The drawing under review shows one solid part. Ordinate dimensions are in mm from its lowest x, y, z. A direction names the side the tool comes from. Give positions to 0.01 mm unless a question says otherwise; leave off trailing zeros. Order: outer loops, then holes, each group sorted by start corner. A loop starts at its lowest first (then second) coordinate and runs counter-clockwise, first axis right, second up. Notation, with made-up numbers: (45.5, -33) -> (57.5, -33) arc R20 cw to (57.5, 3) -> close; hole circle Ø3 at (40, 50). An arc over 180 degrees is marked (long way). One line per item, written item: value. Start each with the question number.
1) Consider section A-A (z = 3.25). State the section outline as (x, y) points, plus the area to 3 significant figures.
2) Consider section C-C (z = 17.75). State the section outline as (x, y) points, plus the area to 3 significant figures.
3) Tool access review of the marked faces 1, 2 and 3: name each direction out of +Z, -Z, +X, -X, +Y, -Y from which nothing blocks a thin tool from reaching the whole face with its end or side.
4) Consider section B-B (z = 7). State the section outline as (x, y) points, plus the area to 3 significant figures.
5) For pin 1 (2 mm diameter, centred on y = 2, z = 9.5, fed in from -X), flat-tipped, find the tip position at first contact; note if it passes through.
6) Wall thickness on line 1 along Z through (x, y) = (1.25, 3.25); line 2 along Z through (x, y) = (0.8, 1.9); line 3 along Z through (x, y) = (4, 3.4): over which ranges is each line inside the solid? List them lowest first. Write a range as from..to.
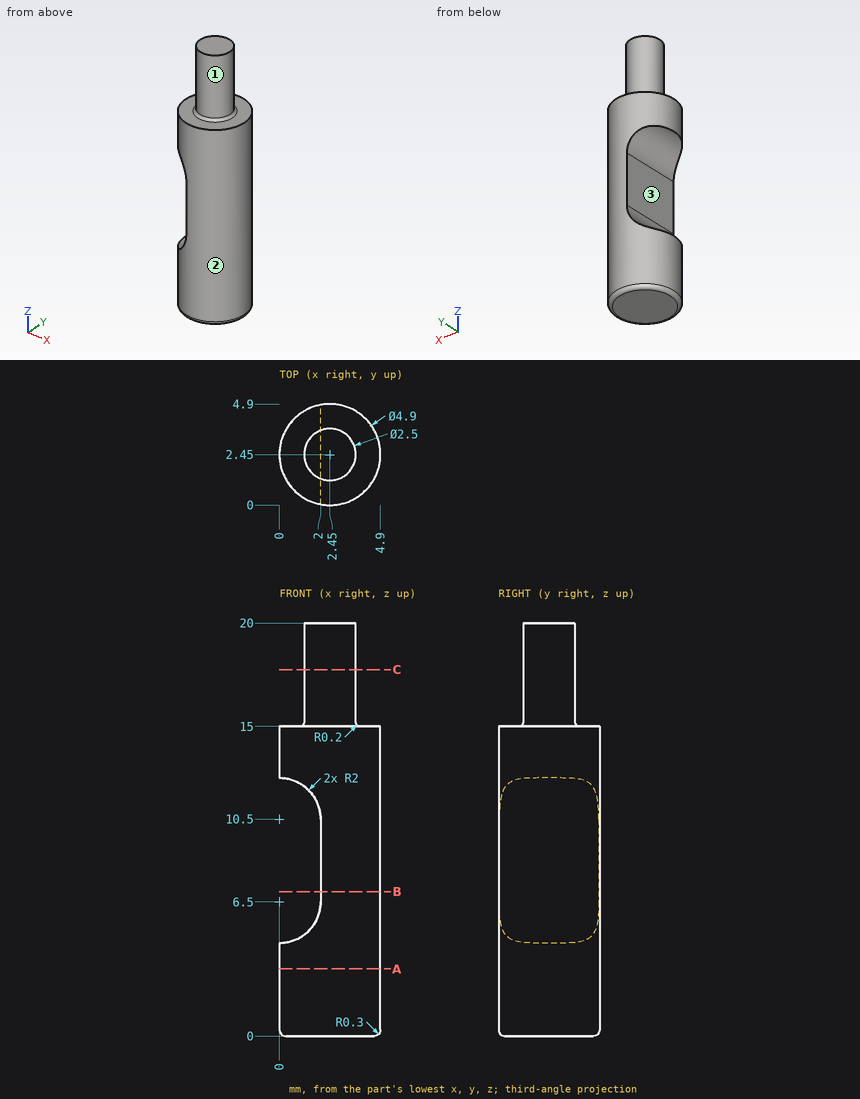
Checked values:
1. outline: circle Ø4.9 at (2.45, 2.45)
1. area: 18.9 mm^2
2. outline: circle Ø2.5 at (2.45, 2.45)
2. area: 4.91 mm^2
3. face 1: +Z
3. face 2: +Z, -Z
3. face 3: -X, +Y, -Y
4. outline: (2, 0.04) arc R2.45 ccw (long way) to (2, 4.86) -> close
4. area: 11.6 mm^2
5. pin 1: stops at x = 2
6. line 1: z = 0..4.94, 12.06..15
6. line 2: z = 0..4.67, 12.33..15
6. line 3: z = 0..15
